from build123d import *

# Parameters (mm, degrees)
SKETCH1_W           = 100
SKETCH1_H           = 100
BOSS_EXTRUDE1_DEPTH = 100
SKETCH2_W           = 80
SKETCH2_H           = 80
CUT_EXTRUDE1_DEPTH  = 80
SKETCH3_R           = 10
CUT_EXTRUDE2_DEPTH  = 20
SKETCH3_5_R         = 20
SKETCH3_5_R_2       = 10
BOSS_EXTRUDE3_DEPTH = 30


with BuildPart() as part:
    # Sketch1 → Boss-Extrude1 (new body)
    with BuildSketch(Plane.XY):
        with Locations((50, 50)):
            Rectangle(SKETCH1_W, SKETCH1_H)
    extrude(amount=BOSS_EXTRUDE1_DEPTH)

    # Sketch2 → Cut-Extrude1 (cut)
    with BuildSketch(Plane(origin=(0, 100, 0), x_dir=(1, 0, 0), z_dir=(0, 1, 0))):
        with Locations((60, -60)):
            Rectangle(SKETCH2_W, SKETCH2_H)
    extrude(amount=-CUT_EXTRUDE1_DEPTH, mode=Mode.SUBTRACT)

    # Sketch3 → Cut-Extrude2 (cut)
    with BuildSketch(Plane.XY.offset(20)):
        with Locations((60, 60)):
            Circle(SKETCH3_R)
    extrude(amount=-CUT_EXTRUDE2_DEPTH, mode=Mode.SUBTRACT)

    # Sketch3_5 → Boss-Extrude3 (add)
    with BuildSketch(Plane.XY.offset(20)):
        with Locations((60, 60)):
            Circle(SKETCH3_5_R)
        with Locations((60, 60)):
            Circle(SKETCH3_5_R_2, mode=Mode.SUBTRACT)
    extrude(amount=BOSS_EXTRUDE3_DEPTH)


solid = part.part
Work out the finished part from the listing and answer in its coordinate system (mm). A direction names the side the tool comes from. Give positions to 0.01 mm unless a question says otherwise; leave off trailing zeros. Loops run counter-clockwise (first coordinate to the right, second up) from the corner with the lowest first, then second, coordinate; pieces in that order, holes last. Notation, with made-up numbers: (-1, 87.25) - (5, 87.25) arc R10 cw to (5, 103.25) - close; hole circle Ø7 at (38, 66). An arc over 180 degrees is marked (long way). Answer in a Markdown table with one row per item. Add a question column.
Q1. The part is cut by section A-A (x = 60). Determine the outline of the cut face in (y, z).
Q2. Determine the mould class of faces 1 (the flat face through (27, 17, 100)), 2 (the flat face through (50.6, 78.3, 20)), 3 (the flat face through (100, 27, 16)), 4 (the flat face through (20, 61, 61)) for opening direction X: released by +X, released by -X, zero draft, split by the parting line, or undercut.
Q3. The part is cut by section B-B (z = 35.5). Determine the outline of the cut face in (x, y), and give its area (3 significant figures).
Q4. Each of these flat-tipped pins is pushed along its axis until it touches: P1, Ø8, axis at x = 35, z = 84.5, coming from the +Y side; P2, Ø1.5, axis at x = 34, y = 55.5, coming from the +Z side; P3, Ø18, axis at x = 60, y = 60, coming from the +Z side; P4, Ø8, axis at y = 73, z = 32.5, coming from the +X side. Where does it stop, or does it pass through?
Q5. Consider line 1 along Y through (x, z) = (60, 24.5); line 2 along Y through (x, z) = (60, 18); line 3 along X through (y, z) = (93.5, 27). Determine where each line is inside the solid, lowest interval first.
Q6. A tool of negligible diameter and unlimited length cuts with its end or side. For faces 5 (the flat face through (51, 65, 50)), 6 (the flat face through (59, 20, 59)), 7 (the cylindrical face through (69.229, 42.257, 34.79)), 8 (the flat face through (0, 49, 49)), 9 (the flat face through (27, 100, 16)), from which of +Z, -Z, +X, -X, +Y, -Y can it reach the whole face along a straight path? Write none if from no direction.
Q7. The part is cut by section D-D (z = 15.5). Determine the outline of the cut face in (x, y), and give its area (3 significant figures).
Solution:
| question | item | result |
|---|---|---|
| 1 | outline | (0, 0) - (50, 0) - (50, 50) - (40, 50) - (40, 20) - (20, 20) - (20, 100) - (0, 100) - close; (70, 0) - (100, 0) - (100, 20) - (80, 20) - (80, 50) - (70, 50) - close |
| 2 | face 1 | zero draft |
| 2 | face 2 | undercut |
| 2 | face 3 | released by +X |
| 2 | face 4 | undercut |
| 3 | outline | (0, 0) - (100, 0) - (100, 20) - (20, 20) - (20, 100) - (0, 100) - close; circle Ø40 at (60, 60); hole circle Ø20 at (60, 60) |
| 3 | area | 4,540 mm² |
| 4 | P1 | stops at y = 20 |
| 4 | P2 | stops at z = 20 |
| 4 | P3 | passes through |
| 4 | P4 | stops at x = 77.86 |
| 5 | line 1 | y = 0 to 20, 40 to 50, 70 to 80 |
| 5 | line 2 | y = 0 to 50, 70 to 100 |
| 5 | line 3 | x = 0 to 20 |
| 6 | face 5 | +Z, +X, +Y |
| 6 | face 6 | +Z, +X |
| 6 | face 7 | +Z |
| 6 | face 8 | +Z, -Z, -X, +Y, -Y |
| 6 | face 9 | +Z, -Z, +X, -X, +Y |
| 7 | outline | (0, 0) - (100, 0) - (100, 100) - (0, 100) - close; hole circle Ø20 at (60, 60) |
| 7 | area | 9,690 mm² |
